Build history of the part. All positions in model axes, mm. A direction names the side the tool comes from. Round coordinates to 2 decimals unless told otherwise and drop trailing zeros. Write each loop counter-clockwise with the first axis right and the second up, starting at its lowest first coordinate (ties: lowest second). Pieces come first, ordered by that corner, then holes. Notation, with made-up numbers: (-29.5, 66) - (24.5, 66) arc R22 ccw to (24.5, 82) - close; hole circle Ø11 at (66, 5). An arc over 180 degrees is marked (long way). Write each question's results on one line, items separated by ' | '.
from build123d import *

# Parameters (mm, degrees)
BOSS_EXTRUDE1_DEPTH = 40
SKETCH5_R           = 25
CUT_EXTRUDE1_DEPTH  = 20
SKETCH6_R           = 16
CUT_EXTRUDE2_DEPTH  = 20
SKETCH7_R           = 7
CUT_EXTRUDE3_DEPTH  = 25
CIRPATTERN1_COUNT   = 6
SKETCH8_R           = 12
CUT_EXTRUDE4_DEPTH  = 15
CIRPATTERN2_COUNT   = 6
CUT_EXTRUDE5_DEPTH  = 10
SKETCH13_R          = 10
CUT_EXTRUDE10_DEPTH = 20


with BuildPart() as part:
    # Sketch3 → Boss-Extrude1 (new body)
    with BuildSketch(Plane(origin=(0, 0, 0), x_dir=(1, 0, 0), z_dir=(0, 1, 0))):
        with BuildLine():
            Line((0, 0), (184, 0))
            Line((184, 0), (184, 250))
            ThreePointArc((184, 250), (92, 342), (0, 250))
            Line((0, 250), (0, 0))
        make_face()
    extrude(amount=BOSS_EXTRUDE1_DEPTH)

    # Sketch5 → Cut-Extrude1 (cut)
    with BuildSketch(Plane(origin=(0, 40, 0), x_dir=(1, 0, 0), z_dir=(0, 1, 0))):
        with Locations((92, 250)):
            Circle(SKETCH5_R)
    extrude(amount=-CUT_EXTRUDE1_DEPTH, mode=Mode.SUBTRACT)

    # Sketch6 → Cut-Extrude2 (cut)
    with BuildSketch(Plane.XZ):
        with Locations((92, -250)):
            Circle(SKETCH6_R)
    extrude(amount=-CUT_EXTRUDE2_DEPTH, mode=Mode.SUBTRACT)

    # Sketch7 → Cut-Extrude3 (cut)
    with BuildSketch(Plane(origin=(0, 40, 0), x_dir=(1, 0, 0), z_dir=(0, 1, 0))):
        with Locations((92, 328)):
            Circle(SKETCH7_R)
    cut_extrude3 = extrude(amount=-CUT_EXTRUDE3_DEPTH, mode=Mode.SUBTRACT)

    # CirPattern1: Cut-Extrude3 ×6 about axis
    cirpattern1_axis = Axis((92, 0, -250), (0, 1, 0))
    for i in range(1, CIRPATTERN1_COUNT):
        add(cut_extrude3.rotate(cirpattern1_axis, i * 360 / CIRPATTERN1_COUNT), mode=Mode.SUBTRACT)

    # Sketch8 → Cut-Extrude4 (cut)
    with BuildSketch(Plane.XZ):
        with Locations((92, -328)):
            Circle(SKETCH8_R)
    cut_extrude4 = extrude(amount=-CUT_EXTRUDE4_DEPTH, mode=Mode.SUBTRACT)

    # CirPattern2: Cut-Extrude4 ×6 about axis
    cirpattern2_axis = Axis((92, 0, -250), (0, 1, 0))
    for i in range(1, CIRPATTERN2_COUNT):
        add(cut_extrude4.rotate(cirpattern2_axis, i * 360 / CIRPATTERN2_COUNT), mode=Mode.SUBTRACT)

    # Sketch9 → Cut-Extrude5 (cut)
    with BuildSketch(Plane(origin=(0, 40, 0), x_dir=(1, 0, 0), z_dir=(0, 1, 0))):
        with BuildLine():
            Line((36, 24), (148, 24))
            ThreePointArc((148, 24), (156.485281374, 27.514718626), (160, 36))
            Line((160, 36), (160, 132.420765027))
            ThreePointArc((160, 132.420765027), (156.485281374, 140.906046402), (148, 144.420765027))
            ThreePointArc((148, 144.420765027), (92, 128.056374228), (36, 144.420765027))
            ThreePointArc((36, 144.420765027), (27.514718626, 140.906046402), (24, 132.420765027))
            Line((24, 132.420765027), (24, 36))
            ThreePointArc((24, 36), (27.514718626, 27.514718626), (36, 24))
        make_face()
    cut_extrude5 = extrude(amount=-CUT_EXTRUDE5_DEPTH, mode=Mode.SUBTRACT)

    # Mirror1: Cut-Extrude5 across plane
    add(cut_extrude5.mirror(Plane.ZX.offset(20)), mode=Mode.SUBTRACT)

    # Sketch13 → Cut-Extrude10 (cut)
    with BuildSketch(Plane.XY):
        with Locations((32, 20)):
            Circle(SKETCH13_R)
        with Locations((152, 20)):
            Circle(SKETCH13_R)
    extrude(amount=-CUT_EXTRUDE10_DEPTH, mode=Mode.SUBTRACT)


solid = part.part
(1) Flat gauge pins, fed straight in: pin 1 Ø12 at (x, y) = (65, 29) entering from -Z; pin 2 Ø8.5 at (x, z) = (159.55, -211) entering from -Y; pin 3 Ø6 at (x, y) = (150, 25) entering from +Z; pin 4 Ø5 at (x, y) = (97.5, 4) entering from -Z. Where does each tip first touch, or does it go through?
Worked answers:
pin 1: stops at z = -339.57 | pin 2: passes through | pin 3: stops at z = -20 | pin 4: stops at z = -341.95
(2) Slice it at A-A, the plane z = -289. Write the cut outline in (x, y), and give its area (3 significant figures).
Worked answers:
outline: (8.68, 0) - (12.45, 0) - (12.45, 15) - (17.45, 15) - (17.45, 40) - (8.68, 40) - close; (31.45, 15) - (36.45, 15) - (36.45, 0) - (147.55, 0) - (147.55, 15) - (152.55, 15) - (152.55, 40) - (31.45, 40) - close; (166.55, 15) - (171.55, 15) - (171.55, 0) - (175.32, 0) - (175.32, 40) - (166.55, 40) - close | area: 5,250 mm2
(3) Two-plate mould, pull along Z, no slides. Class faces 5 (the flat face through (91, 10, -85)), 6 (the flat face through (91, 20, 0)), 7 (the cylindrical face through (22.933, 27.675, -204.166)), 8 (the cylindrical face through (161.237, 16.17, -9.86)): released by +Z, released by -Z, zero draft, split by the parting line, or undercut.
Worked answers:
face 5: undercut | face 6: released by +Z | face 7: undercut | face 8: zero draft
(4) Tool access for faces 1 (the cylindrical face through (21.2, 27.7, -295.2)), 2 (the flat face through (32, 20, -20)), 3 (the cylindrical face through (156.39, 4.93, -27.42)), 4 (the cylindrical face through (88.745, 30.14, -274.787)): list every direction of +Z, -Z, +X, -X, +Y, -Y with a clear straight run to the whole face (end or side of a thin tool).
Worked answers:
face 1: +Y, -Y | face 2: +Z | face 3: -Y | face 4: +Y
(5) Drill centre lines: probe 1 along Z at (x, y) = (92, 31.5); probe 2 along Z at (x, y) = (92, 3.5); probe 3 along Z at (x, y) = (92, 29.25). Where is each one in solid material? Low to high. Write a range as [from, to].
Worked answers:
probe 1: z = [-342, -335], [-321, -275], [-225, -179], [-165, -128.06], [-24, 0] | probe 2: z = [-342, -340], [-316, -266], [-234, -184], [-160, -128.06], [-24, 0] | probe 3: z = [-342, -335], [-321, -275], [-225, -179], [-165, 0]
(6) Slice it at B-B, the plane y = 35.5. State how many separate pieces and enclosed holes the cut face has, and give its area (3 significant figures).
Worked answers:
separate pieces: 1 | enclosed holes: 8 | area: 41,400 mm2
(7) Slice it at C-C, the plane z = -240. Write the cut outline in (x, y), and give its area (3 significant figures).
Worked answers:
outline: (0, 0) - (79.51, 0) - (79.51, 20) - (69.09, 20) - (69.09, 40) - (0, 40) - close; (104.49, 0) - (184, 0) - (184, 40) - (114.91, 40) - (114.91, 20) - (104.49, 20) - close | area: 5,940 mm2
